Check sheet for the modelled part. Datum: model origin and axes. Units: mm. A direction names the side the tool comes from. Give positions to 0.01 mm unless a question says otherwise; leave off trailing zeros. Loops run counter-clockwise (first coordinate to the right, second up) from the corner with the lowest first, then second, coordinate; pieces in that order, holes last.
```python
from build123d import *

# Parameters (mm, degrees)
BOSS_EXTRUDE1_DEPTH           = 10
FILLET1_R                     = 3
CUT_EXTRUDE1_DEPTH            = 55.386
CHAMFER1_SIZE                 = 1.5
MIRROR3_START                 = -3.745316975
MIRROR3_DEPTH                 = 4.272002108
CSK_FOR_M4_SFHCS1_D           = 4
CSK_FOR_M4_SFHCS1_DEPTH       = 6.4
CSK_FOR_M4_SFHCS1_CSINK_D     = 6
CSK_FOR_M4_SFHCS1_CSINK_ANGLE = 90
CSK_FOR_M4_SFHCS2_D           = 4
CSK_FOR_M4_SFHCS2_CSINK_D     = 6
CSK_FOR_M4_SFHCS2_CSINK_ANGLE = 90
SKETCH7_R                     = 1.5
CUT_EXTRUDE2_DEPTH            = 24
SKETCH8_R                     = 10.5
CUT_EXTRUDE3_DEPTH            = 15
CHAMFER2_SIZE                 = 2


# Read off the part's stored shape, not the designer's step: Mirror3
with BuildPart() as part:
    # Sketch1 → Boss-Extrude1 (new body)
    with BuildSketch(Plane(origin=(0, 0, 0), x_dir=(1, 0, 0), z_dir=(0, 1, 0))):
        with BuildLine():
            Line((-35.25, 0), (-35.25, -6.4))
            Line((-35.25, -6.4), (-22.25, -6.4))
            ThreePointArc((-22.25, -6.4), (-20.128679656, -7.278679656), (-19.25, -9.4))
            Line((-19.25, -9.4), (-19.25, -28.6))
            ThreePointArc((-19.25, -28.6), (-20.128679656, -30.721320344), (-22.25, -31.6))
            Line((-22.25, -31.6), (-35.25, -31.6))
            Line((-35.25, -31.6), (-35.25, -38))
            Line((-35.25, -38), (-5.75, -38))
            ThreePointArc((-5.75, -38), (-5.289009014, -37.946146786), (-4.852843875, -37.787487311))
            Line((-4.852843875, -37.787487311), (-0.384125597, -35.544596998))
            ThreePointArc((-0.384125597, -35.544596998), (0.230625744, -35.066359782), (0.616084961, -34.389564956))
            Line((0.616084961, -34.389564956), (1.30066574, -32.33582167))
            ThreePointArc((1.30066574, -32.33582167), (2.028611742, -31.34579265), (3.198032424, -30.968276939))
            Line((3.198032424, -30.968276939), (32.698032424, -30.968276939))
            ThreePointArc((32.698032424, -30.968276939), (33.642903174, -31.205546312), (34.363585035, -31.861057674))
            Line((34.363585035, -31.861057674), (35.193999483, -33.110222133))
            ThreePointArc((35.193999483, -33.110222133), (35.866740637, -33.73918414), (36.750000973, -34.000000252))
            Line((36.750000973, -34.000000252), (52.750000973, -34.000000252))
            Line((52.750000973, -34.000000252), (52.750000973, -4.000000252))
            Line((52.750000973, -4.000000252), (38.13600074, -4.000000252))
            ThreePointArc((38.13600074, -4.000000252), (36.996810987, -3.643851433), (36.263342318, -2.702246958))
            Line((36.263342318, -2.702246958), (35.25, 0))
            Line((35.25, 0), (-35.25, 0))
        make_face()
    extrude(amount=BOSS_EXTRUDE1_DEPTH)

    # Fillet1
    fillet1_edges = [part.edges().sort_by_distance(p)[0] for p in [
        (52.750000973, 0, 19.000000252),
        (-35.25, 0, 34.8),
        (-35.25, 0, 3.2),
        (-35.25, 10, 34.8),
        (52.750000973, 10, 19.000000252),
        (-35.25, 10, 3.2),
    ]]
    fillet(fillet1_edges, radius=FILLET1_R)

    # Sketch2 → Cut-Extrude1 (cut)
    with BuildSketch(Plane(origin=(38.13600074, 0, 0), x_dir=(0, 0, -1), z_dir=(1, 0, 0))):
        Polygon((-4.000000252, 10), (0, 10), (0, 8.5), align=None)
    extrude(amount=-CUT_EXTRUDE1_DEPTH, mode=Mode.SUBTRACT)

    # Chamfer1
    # the kernel refuses this chamfer: 1.5 mm, written as the material it adds along each edge
    with BuildSketch(Plane(origin=(-17.24999926, 7.145532803, -3.611912754), x_dir=(-0.027495876610586757, 0.9359751746095561, -0.35099066837171944), z_dir=(0, 0.3511234221997007, 0.9363291848398034))) as chamfer1_piece_1_section:
        Polygon((CHAMFER1_SIZE * 0.999621916911, -CHAMFER1_SIZE * 0.0274958766106), (-CHAMFER1_SIZE * 0.0274958766106, -CHAMFER1_SIZE * 0.999621916911), (0, 0), align=None)
    chamfer1_piece_1 = extrude(amount=11.987051072, mode=Mode.PRIVATE)
    chamfer1_piece_1 = split(chamfer1_piece_1, bisect_by=Plane(origin=(-16.68097762, 9.443284972, 0), z_dir=(0, 0, 1)), keep=Keep.TOP, mode=Mode.PRIVATE)
    chamfer1_piece_1 = split(chamfer1_piece_1, bisect_by=Plane(origin=(-16.68097762, 10, 1.484573502), z_dir=(0, -1, 0)), keep=Keep.TOP, mode=Mode.PRIVATE)
    add(chamfer1_piece_1)

    # Mirror3 outline → Mirror3 (cut)
    with BuildSketch(Plane(origin=(0, 0, 0), x_dir=(1, 0, 0), z_dir=(0, 0.3511234221997011, -0.9363291848398033)).offset(MIRROR3_START)):
        Polygon((-15.74999926, -1.404493777), (40, -1.404493777), (40, 2), (-19, 2), (-19, 1.845506963), align=None)
    extrude(amount=MIRROR3_DEPTH, mode=Mode.SUBTRACT)

    # CSK for M4 SFHCS1
    with Locations(Plane.XY.offset(6.4)):
        with Locations((-30.25, 5)):
            csk_for_m4_sfhcs1 = CounterSinkHole(CSK_FOR_M4_SFHCS1_D / 2, CSK_FOR_M4_SFHCS1_CSINK_D / 2, depth=CSK_FOR_M4_SFHCS1_DEPTH, counter_sink_angle=CSK_FOR_M4_SFHCS1_CSINK_ANGLE)

    # Mirror1: CSK for M4 SFHCS1 across plane
    add(csk_for_m4_sfhcs1.mirror(Plane.XY.offset(19)), mode=Mode.SUBTRACT)

    # CSK for M4 SFHCS2 (through all)
    with Locations(Plane.XY.offset(34.000000252)):
        with Locations((46.750000973, 5)):
            csk_for_m4_sfhcs2 = CounterSinkHole(CSK_FOR_M4_SFHCS2_D / 2, CSK_FOR_M4_SFHCS2_CSINK_D / 2, counter_sink_angle=CSK_FOR_M4_SFHCS2_CSINK_ANGLE)

    # Mirror2: CSK for M4 SFHCS2 across plane
    add(csk_for_m4_sfhcs2.mirror(Plane.XY.offset(19)), mode=Mode.SUBTRACT)

    # Sketch7 → Cut-Extrude2 (cut)
    with BuildSketch(Plane(origin=(0, 0, 0), x_dir=(-1, 0, 0), z_dir=(0, 0, -1))):
        with Locations((-31.25, 5)):
            Circle(SKETCH7_R)
        with Locations((-23.75, 5)):
            Circle(SKETCH7_R)
        with Locations((-16.25, 5)):
            Circle(SKETCH7_R)
        with Locations((-8.75, 5)):
            Circle(SKETCH7_R)
        with Locations((-1.25, 5)):
            Circle(SKETCH7_R)
        with Locations((6.25, 5)):
            Circle(SKETCH7_R)
        with Locations((13.75, 5)):
            Circle(SKETCH7_R)
    extrude(amount=-CUT_EXTRUDE2_DEPTH, mode=Mode.SUBTRACT)

    # Sketch8 → Cut-Extrude3 (cut)
    with BuildSketch(Plane(origin=(52.750000973, 0, 0), x_dir=(0, 0, -1), z_dir=(1, 0, 0))):
        with Locations((-19.000000252, 18.5)):
            Circle(SKETCH8_R)
        with Locations((-19.000000252, -8.5)):
            Circle(SKETCH8_R)
    extrude(amount=-CUT_EXTRUDE3_DEPTH, mode=Mode.SUBTRACT)

    # Chamfer2
    # the kernel refuses this chamfer: 2 mm, written as the material it adds along each edge
    # the kernel refuses this chamfer: 2 mm, written as the material it takes off along each edge
    with BuildSketch(Plane(origin=(37.750000973, 10, 7.692220273), x_dir=(-0.9996219169112968, 0.02749587661058651, 0), z_dir=(0, 0, 1))) as chamfer2_2_piece_1_section:
        Polygon((CHAMFER2_SIZE * 0.999621916911, CHAMFER2_SIZE * 0.0274958766106), (-CHAMFER2_SIZE * 0.0274958766106, CHAMFER2_SIZE * 0.999621916911), (0, 0), align=None)
    chamfer2_2_piece_1 = extrude(amount=22.615559958, mode=Mode.PRIVATE)
    chamfer2_2_piece_1 = chamfer2_2_piece_1 & Plane(origin=(37.038023767, 18.5, 19.000000252), x_dir=(0, 0, -1), z_dir=(1, 0, 0)) * Cylinder(10.5, 54, mode=Mode.PRIVATE)
    add(chamfer2_2_piece_1, mode=Mode.SUBTRACT)
    with BuildSketch(Plane(origin=(37.750000973, 0, 30.307780231), x_dir=(-0.9996219169112968, -0.02749587661058639, 0), z_dir=(0, 0, -1))) as chamfer2_2_piece_2_section:
        Polygon((CHAMFER2_SIZE * 0.999621916911, CHAMFER2_SIZE * 0.0274958766106), (-CHAMFER2_SIZE * 0.0274958766106, CHAMFER2_SIZE * 0.999621916911), (0, 0), align=None)
    chamfer2_2_piece_2 = extrude(amount=22.615559958, mode=Mode.PRIVATE)
    chamfer2_2_piece_2 = chamfer2_2_piece_2 & Plane(origin=(37.038023767, -8.5, 19.000000252), x_dir=(0, 0, -1), z_dir=(1, 0, 0)) * Cylinder(10.5, 54, mode=Mode.PRIVATE)
    add(chamfer2_2_piece_2, mode=Mode.SUBTRACT)


solid = part.part
```
(1) Gauge pin test, flat ends, axial feed: pin 1 Ø3 at (x, y) = (-30.25, 5) entering from +Z; pin 2 Ø2 at (x, y) = (-0.5, 1) entering from +Z; pin 3 Ø4 at (x, y) = (-13.75, 5) entering from -Z; pin 4 Ø2 at (y, z) = (4.5, 15.5) entering from -X. Record the tip position at first contact, or that the pin passes through.
(2) Access from +Z, -Z, +X, -X, +Y, -Y to the whole of each face (thin tool, end or side, straight path). Record for faces 4 (the face through (17.75, 5.07, 11.83)), 5 (the face through (36.51, 0.76, 19.09)), 6 (the face through (18, 5, 30.968)).
(3) Section check D-D on x = -13.75. Record the boundary of the cut face in (y, z), plus the area to 3 significant figures.
(4) Release check for a two-part mould opening along Y. For faces 1 (the face through (-2.65, 4.93, 36.68)), 2 (the face through (25.25, 5.07, 11.83)), 3 (the face through (44, 8, 19)) record: pulls with the +Y half, pulls with the -Y half, needs draft (parallel to the pull), parting line crosses it, or undercut.
(5) Section check B-B on x = 31.25. Record the boundary of the cut face in (y, z), plus the area to 3 significant figures.
(6) Section check A-A on x = -30.25. Record the boundary of the cut face in (y, z), plus the area to 3 significant figures.
(7) Section check C-C on y = 5. Give the number of separate pieces and of enclosed holes in the cut face, plus the area to 3 significant figures.
(8) Material ranges on line 1 (Z direction, x = -25.5, y = 5.75); line 2 (X direction, y = 5, z = 24.25); line 3 (Y direction, x = -6.25, z = 9.75), recorded low to high.
Computed values:
1. pin 1: passes through
1. pin 2: stops at z = 36.1
1. pin 3: stops at z = 0
1. pin 4: stops at x = -19.25
2. face 4: -Z
2. face 5: +X, -Y
2. face 6: +Z, +Y, -Y
3. outline: (0, 4) - (1.5, 0) - (3.5, 0) - (3.5, 24) - (6.5, 24) - (6.5, 0) - (8.5, 0) - (10, 4) - (10, 38) - (0, 38) - close
3. area: 302 mm2
4. face 1: needs draft
4. face 2: undercut
4. face 3: pulls with the +Y half
5. outline: (0, 4) - (1.5, 0) - (3.5, 0) - (3.5, 24) - (6.5, 24) - (6.5, 0) - (8.5, 0) - (10, 4) - (10, 30.97) - (0, 30.97) - close
5. area: 232 mm2
6. outline: (0, 0) - (3, 0) - (3, 5.4) - (2, 6.4) - (0, 6.4) - close; (0, 31.6) - (2, 31.6) - (3, 32.6) - (3, 38) - (0, 38) - close; (7, 0) - (10, 0) - (10, 6.4) - (8, 6.4) - (7, 5.4) - close; (7, 32.6) - (8, 31.6) - (10, 31.6) - (10, 38) - (7, 38) - close
6. area: 74.8 mm2
7. separate pieces: 4
7. enclosed holes: 0
7. area: 1,880 mm2
8. line 1: z = 0 to 6.4, 31.6 to 38
8. line 2: x = -19.25 to 44.75, 48.75 to 52.75
8. line 3: y = 0 to 3.5, 6.5 to 10
